Could you check a few things on this model? Use its own coordinates, in mm. A direction names the side the tool comes from. Give positions to 0.01 mm unless a question says otherwise; leave off trailing zeros. Order: outer loops, then holes, each group sorted by start corner. A loop starts at its lowest first (then second) coordinate and runs counter-clockwise, first axis right, second up. Notation, with made-up numbers: (59, 79) -> (81, 79) arc R30 cw to (81, 115) -> close; hole circle Ø5 at (-39.75, 5). An arc over 180 degrees is marked (long way). Use one line per item in the form item = value. Start each with the question number.
Autodesk Fusion 360 part; units mm, degrees
sketch "Sketch1" plane through (0, 0, 0) normal (0, 1, 0) x (1, 0, 0)
  line L0 (0, 0) -> (-4.8, 0)
  line L1 (-4.8, 0) -> (-4.8, -10)
  line L2 (-4.8, -10) -> (0, -10)
  line L3 (0, -10) -> (0, -30)
  line L4 (0, -30) -> (4.8, -30)
  line L5 (4.8, -30) -> (4.8, 0)
  line L6 (4.8, 0) -> (0, 0)
  line L7 (0, 0) -> (0, -10) construction
  line L8 (-10.4, 10) -> (34.8, 10)
  line L9 (9.8, -25) -> (14.6, -25) construction
  line L10 (14.6, -25) -> (14.6, -20.2) construction
  line L11 (14.6, -20.2) -> (9.8, -20.2) construction
  line L12 (9.8, -20.2) -> (9.8, -25) construction
  line L13 (9.8, -22.6) -> (29.8, -22.6) construction
  line L14 (12.2, -20.2) -> (12.2, -40.2) construction
  circle A0 centre (12.2, -22.6) radius 3.3941
  arc A1 (31.3, -22.6) -> (12.2, -41.7) centre (12.2, -22.6) ccw construction
  arc A2 (12.2, -41.7) -> (31.3, -22.6) centre (12.2, -22.6) ccw
  arc A3 (28.3, -22.6) -> (12.2, -38.7) centre (12.2, -22.6) ccw construction
  arc A4 (12.2, -38.7) -> (28.3, -22.6) centre (12.2, -22.6) ccw
  arc A5 (12.2, -38.7) -> (12.2, -41.7) centre (12.2, -40.2) ccw
  arc A6 (12.2, -41.7) -> (12.2, -38.7) centre (12.2, -40.2) ccw construction
  arc A7 (31.3, -22.6) -> (28.3, -22.6) centre (29.8, -22.6) ccw
  arc A8 (28.3, -22.6) -> (31.3, -22.6) centre (29.8, -22.6) ccw construction
  circle A9 centre (12.2, -40.2) radius 5 construction
  line L15 (-10.4, 10) -> (-10.4, -22.6)
  arc A10 (12.2, -45.2) -> (12.2, -45.2) centre (12.2, -22.6) ccw
  line L16 (34.8, -22.6) -> (34.8, 10)
  line L17 (9.8, -25) -> (4.8, -25) construction
  arc A11 (34.8, -22.6) -> (-10.4, -22.6) centre (12.2, -22.6) ccw construction
  arc A12 (-10.4, -22.6) -> (12.2, -45.2) centre (12.2, -22.6) ccw
  arc A13 (12.2, -45.2) -> (34.8, -22.6) centre (12.2, -22.6) ccw
  point P0 (12.2, -20.2)
  point P1 (9.8, -22.6)
  point P2 (12.2, -22.6)
  dimension "d23" = 4.8
  dimension "d24" = 10
  dimension "d26" = 4.8
  dimension "d27" = 10
  dimension "d31" = 4.8
  dimension "d32" = 4.8
  dimension "d33" = 20
  dimension "d34" = 20
  dimension "d35" = 3
  dimension "d36" = 3
  dimension "d37" = 10
  dimension "d38" = 30
  dimension "d40" = 5
  dimension "d41" = 5
extrude "Extrude1" add sketch "Sketch1" along normal blind 4.8 contours L0 L1 L5 L6 L8 L15 A10 L16 | L1 L2 L3 L4 L5 A10 A12 A13
(1) Imagine slicing it at A-A (z = 16.5). Write out the boundary of the cut face in (x, y).
(2) Imagine slicing it at C-C (x = 27). Write out the boundary of the cut face in (y, z), plus the area to 3 significant figures.
(3) Please list where these lines run through material, in increasing order: probe 1 along X at (y, z) = (2, 22.6); probe 2 along Z at (x, y) = (12.2, 2.65); probe 3 along X at (y, z) = (2.3, 7.5).
(4) Which directions (+Z, -Z, +X, -X, +Y, -Y) give clear straight access to the entire face, cutting with the end or side of a thin tool? Please do faces 1 (the cylindrical face through (25.85, 2.37, 35.96)), 2 (the flat face through (-10.4, 2, 6)).
(5) Imagine slicing it at B-B (y = 3.65). Write out the boundary of the cut face in (x, z).
(6) I'm going to push flat-ended pins straight in: pin 1 Ø2.5 at (x, y) = (-1, 3) entering from +Z; pin 2 Ø1.5 at (x, y) = (-2, 1) entering from +Z. Where does each tip first touch, or does it pass through?
Calculated:
q1.outline = (-10.4, 0) -> (0, 0) -> (0, 4.8) -> (-10.4, 4.8) -> close; (4.8, 0) -> (34.8, 0) -> (34.8, 4.8) -> (4.8, 4.8) -> close
q2.outline = (0, -10) -> (4.8, -10) -> (4.8, 28.94) -> (0, 28.94) -> close; (0, 34.67) -> (4.8, 34.67) -> (4.8, 39.68) -> (0, 39.68) -> close
q2.area = 211 mm2
q3.probe_1 = -10.4 to 0, 4.8 to 8.81, 15.59 to 28.3, 31.3 to 34.8
q3.probe_2 = -10 to 19.21, 25.99 to 38.7, 41.7 to 45.2
q3.probe_3 = -10.4 to -4.8, 4.8 to 34.8
q4.face_1 = +Y, -Y
q4.face_2 = +Z, -Z, -X, +Y, -Y
q5.outline = (-10.4, -10) -> (34.8, -10) -> (34.8, 22.6) arc R22.6 ccw to (-10.4, 22.6) -> close; hole (-4.8, 0) -> (4.8, 0) -> (4.8, 30) -> (0, 30) -> (0, 10) -> (-4.8, 10) -> close; hole circle Ø6.79 at (12.2, 22.6); hole (12.2, 38.7) arc R16.1 cw to (28.3, 22.6) arc R1.5 ccw to (31.3, 22.6) arc R19.1 ccw to (12.2, 41.7) arc R1.5 ccw to start
q6.pin_1 = 41.78
q6.pin_2 = 40.76
